Part print with two shaded views. Sizes in mm from the minimum x, y, z corner. A direction names the side the tool comes from. Round coordinates to 2 decimals unless told otherwise and drop trailing zeros. Loops run counter-clockwise (first coordinate to the right, second up) from the corner with the lowest first, then second, coordinate; pieces in that order, holes last. Notation, with made-up numbers: (-27, 76.5) -> (28, 76.5) arc R19 ccw to (28, 84.5) -> close; hole circle Ø4 at (29.25, 80). An arc over 180 degrees is marked (long way). Use a Markdown table: item, result. Add a question column.
Item 1: Cut at C-C, the plane y = 17.5. List the corners of the cut face in (x, z) (1 decimal), plus the area to 3 significant figures.
Item 2: Cut at D-D, the plane z = 3.5. List the corners of the cut face in (x, y) (1 decimal).
Item 3: Two-plate mould, pull along X, no slides. Class the marked faces 4, 5, 6 and 7: pulls with the +X half, pulls with the -X half, needs draft (parallel to the pull), parting line crosses it, or undercut.
Item 4: Cut at B-B, the plane x = 33.5. List the corners of the cut face in (y, z), plus the area to 3 significant figures.
Item 5: Flat gauge pins, fed straight in: pin 1 (10 mm diameter, centred on y = 5, z = 5.5, fed in from -X); pin 2 (1.5 mm diameter, centred on y = 10.5, z = 7.5, fed in from -X); pin 3 (1.5 mm diameter, centred on x = 29, z = 7.5, fed in from +Y); pin 4 (10 mm diameter, centred on y = 31.5, z = 11.5, fed in from -X). Where does each tip first touch, or does it go through?
Item 6: Which spindle directions (+Z, -Z, +X, -X, +Y, -Y) get a long thin tool onto all of the face, cutting with end or side? Do the marked faces 1, 2 and 3. Say none if no direction does.
Item 7: Cut at A-A, the plane z = 10.5. List the corners of the cut face in (x, y) (1 decimal), plus the area to 3 significant figures.
Item 8: Probe line 1 (Y direction, x = 40.5, z = 16) (1 decimal); line 2 (X direction, y = 13.5, z = 6.5); line 3 (X direction, y = 27.5, z = 8.75). List the from-to ranges inside material, lowest first. Write a range as [from, to].
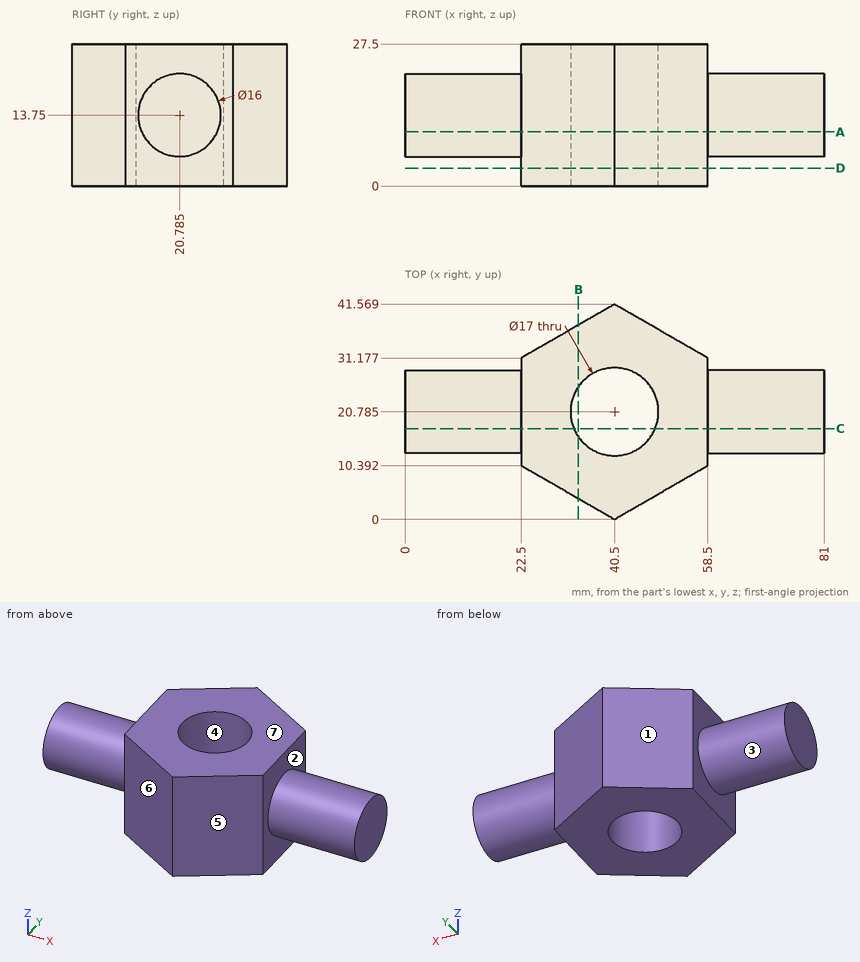
A:
| question | item | result |
|---|---|---|
| 1 | outline | (0, 6.5) -> (22.5, 6.5) -> (22.5, 0) -> (32.7, 0) -> (32.7, 27.5) -> (22.5, 27.5) -> (22.5, 21) -> (0, 21) -> close; (48.3, 0) -> (58.5, 0) -> (58.5, 6.5) -> (81, 6.5) -> (81, 21) -> (58.5, 21) -> (58.5, 27.5) -> (48.3, 27.5) -> close |
| 1 | area | 1,220 mm^2 |
| 2 | outline | (22.5, 10.4) -> (40.5, 0) -> (58.5, 10.4) -> (58.5, 31.2) -> (40.5, 41.6) -> (22.5, 31.2) -> close; hole circle Ø17 at (40.5, 20.8) |
| 3 | face 4 | undercut |
| 3 | face 5 | pulls with the +X half |
| 3 | face 6 | pulls with the -X half |
| 3 | face 7 | needs draft |
| 4 | outline | (4.04, 0) -> (15.96, 0) -> (15.96, 27.5) -> (4.04, 27.5) -> close; (25.61, 0) -> (37.53, 0) -> (37.53, 27.5) -> (25.61, 27.5) -> close |
| 4 | area | 656 mm^2 |
| 5 | pin 1 | stops at x = 23.18 |
| 5 | pin 2 | stops at x = 22.5 |
| 5 | pin 3 | stops at y = 35.36 |
| 5 | pin 4 | stops at x = 0 |
| 6 | face 1 | +Z, -Z, -X, +Y |
| 6 | face 2 | +X |
| 6 | face 3 | -X |
| 7 | outline | (0, 13.5) -> (22.5, 13.5) -> (22.5, 10.4) -> (40.5, 0) -> (58.5, 10.4) -> (58.5, 13.5) -> (81, 13.5) -> (81, 28.1) -> (58.5, 28.1) -> (58.5, 31.2) -> (40.5, 41.6) -> (22.5, 31.2) -> (22.5, 28.1) -> (0, 28.1) -> close; hole circle Ø17 at (40.5, 20.8) |
| 7 | area | 1,550 mm^2 |
| 8 | line 1 | y = [0, 12.3], [29.3, 41.6] |
| 8 | line 2 | x = [22.5, 36.12], [44.88, 58.5] |
| 8 | line 3 | x = [22.5, 35.29], [45.71, 58.5] |
